from build123d import *

# Parameters (mm, degrees)
SKETCH_1_W      = 615
SKETCH_1_H      = 83
SKETCH_1_R      = 2.555
EXTRUDE_1_DEPTH = 4
FILLET_1_R      = 10


with BuildPart() as part:
    # 草图1 → 凸台-拉伸1 (new body)
    with BuildSketch(Plane.XY):
        Rectangle(SKETCH_1_W, SKETCH_1_H)
        with Locations((-298.155, -34.6)):
            Circle(SKETCH_1_R, mode=Mode.SUBTRACT)
        with Locations((-298.155, -21.9)):
            Circle(SKETCH_1_R, mode=Mode.SUBTRACT)
        with Locations((-298.155, -9.2)):
            Circle(SKETCH_1_R, mode=Mode.SUBTRACT)
        with Locations((-298.155, 3.5)):
            Circle(SKETCH_1_R, mode=Mode.SUBTRACT)
        with Locations((-298.155, 16.2)):
            Circle(SKETCH_1_R, mode=Mode.SUBTRACT)
        with Locations(Location((298.155, 16.2, 0), (0, 0, 180))):
            Circle(SKETCH_1_R, mode=Mode.SUBTRACT)
        with Locations(Location((298.155, 3.5, 0), (0, 0, 180))):
            Circle(SKETCH_1_R, mode=Mode.SUBTRACT)
        with Locations(Location((298.155, -9.2, 0), (0, 0, 180))):
            Circle(SKETCH_1_R, mode=Mode.SUBTRACT)
        with Locations(Location((298.155, -21.9, 0), (0, 0, 180))):
            Circle(SKETCH_1_R, mode=Mode.SUBTRACT)
        with Locations(Location((298.155, -34.6, 0), (0, 0, 180))):
            Circle(SKETCH_1_R, mode=Mode.SUBTRACT)
        with Locations((-298.155, 28.9)):
            Circle(SKETCH_1_R, mode=Mode.SUBTRACT)
        with Locations(Location((298.155, 28.9, 0), (0, 0, 180))):
            Circle(SKETCH_1_R, mode=Mode.SUBTRACT)
    extrude(amount=EXTRUDE_1_DEPTH)

    # 圆角1
    fillet_1_edges = [part.edges().sort_by_distance(p)[0] for p in [
        (307.5, -41.5, 2),
        (-307.5, -41.5, 2),
        (-307.5, 41.5, 2),
        (307.5, 41.5, 2),
    ]]
    fillet(fillet_1_edges, radius=FILLET_1_R)


solid = part.part
Verification items for the finished model (mm, model axes). Round coordinates to 2 decimals unless told otherwise and drop trailing zeros. Put each result on its own line as item: value.
1) Material ranges on line 1 (X direction, y = -10.5, z = 2.55); line 2 (X direction, y = -35, z = 2.45); line 3 (X direction, y = 32.5, z = 3), recorded low to high.
Final values:
line 1: x = -307.5 to -300.35, -295.96 to 295.96, 300.35 to 307.5
line 2: x = -306.87 to -300.68, -295.63 to 295.63, 300.68 to 306.87
line 3: x = -307.45 to 307.45
2) Mould release check, pull along Y, two halves, no side actions. Record for faces 1 (the flat face through (-4, 1, 0)), 2 (the cylindrical face through (-304.65, 38.49, 2.03)), 3 (the cylindrical face through (-304.65, -38.49, 2.03)): +Y half, -Y half, draft (parallel to the pull), parting line (faces both ways), or undercut.
Final values:
face 1: draft
face 2: +Y half
face 3: -Y half
3) Depth check by flat-ended pin: pin 1 (8 mm diameter, centred on x = -298.155, y = 3.5, fed in from -Z). Enter the tip coordinate at first touch or a pass-through.
Final values:
pin 1: stops at z = 0
